Autodesk Fusion 360 part; units mm, degrees
sketch "Bottom Access Panel" plane through (0, 0, 0) normal (0, 1, 0) x (1, 0, 0)
  line L0 (0, 0) -> (140, 0)
  line L1 (140, 0) -> (140, -140)
  line L2 (140, -140) -> (0, -140)
  line L3 (0, -140) -> (0, 0)
  dimension "d1" = 140
  dimension "d2" = 140
extrude "Extrude1" add sketch "Bottom Access Panel" along normal blind 6
fillet "Fillet1" radius 8 4 edges at (0, 3, 140) (140, 3, 140) (140, 3, 0) (0, 3, 0)
sketch "Magnet Holes" plane through (0, 0, 0) normal (0, 1, 0) x (1, 0, 0)
  arc A0 (8, 0) -> (0, -8) centre (8, -8) ccw
  line L0 (8, 0) -> (132, 0)
  arc A1 (140, -8) -> (132, 0) centre (132, -8) ccw
  line L1 (140, -8) -> (140, -132)
  arc A2 (132, -140) -> (140, -132) centre (132, -132) ccw
  line L2 (132, -140) -> (8, -140)
  arc A3 (0, -132) -> (8, -140) centre (8, -132) ccw
  line L3 (0, -132) -> (0, -8)
  circle A4 centre (10, -130) radius 2.75
  circle A5 centre (130, -130) radius 2.75
  circle A6 centre (10, -10) radius 2.75
  circle A7 centre (130, -10) radius 2.75
  dimension "d20" = 5.5
  dimension "d21" = 5.5
  dimension "d22" = 5.5
  dimension "d23" = 5.5
  dimension "d24" = 10
  dimension "d25" = 10
  dimension "d26" = 10
  dimension "d27" = 10
  dimension "d28" = 10
  dimension "d29" = 10
  dimension "d30" = 10
  dimension "d31" = 10
extrude "Extrude3" cut sketch "Magnet Holes" along normal blind 1.5 contours A4 | A5 | A6 | A7
equation "mdfThickness = 6 mm"
equation "d4 = mdfThickness"
equation "filletRadius = 8 mm"
equation "d15 = filletRadius"
Part model, mm, in its own coordinate system. A direction names the side the tool comes from. Round coordinates to 2 decimals unless told otherwise and drop trailing zeros. Write each loop counter-clockwise with the first axis right and the second up, starting at its lowest first coordinate (ties: lowest second). Pieces come first, ordered by that corner, then holes.
Item 1: Probe L1, parallel to Z at x = 130, y = 1.15. List the from-to ranges inside material, lowest first.
Results:
L1: z = 0 to 7.25, 12.75 to 127.25, 132.75 to 140
Item 2: Which spindle directions (+Z, -Z, +X, -X, +Y, -Y) get a long thin tool onto all of the face, cutting with end or side? Do faces 1 (the cylindrical face through (137.594, 3.042, 137.719)), 2 (the flat face through (10, 1.5, 10)). Say none if no direction does.
Results:
face 1: +Z, +X, +Y, -Y
face 2: -Y
Item 3: Two-plate mould, pull along X, no slides. Class faces 3 (the flat face through (130, 1.5, 130)), 4 (the cylindrical face through (131.27, 0.74, 127.56)), 5 (the flat face through (140, 3, 69)), 6 (the flat face through (69, 0, 69)): +X half, -X half, draft (parallel to the pull), parting line (faces both ways), or undercut.
Results:
face 3: undercut
face 4: undercut
face 5: +X half
face 6: draft
Item 4: Drop a flat-ended pin along its axis: pin 1 Ø1.6 at (x, z) = (9.5, 9) entering from -Y. Give the stop position or say it passes through.
Results:
pin 1: stops at y = 1.5
Item 5: Cut at B-B, the plane z = 10. Give the cut face in (x, y).
Results:
outline: (0, 0) - (7.25, 0) - (7.25, 1.5) - (12.75, 1.5) - (12.75, 0) - (127.25, 0) - (127.25, 1.5) - (132.75, 1.5) - (132.75, 0) - (140, 0) - (140, 6) - (0, 6) - close
Item 6: Cut at A-A, the plane x = 130. Give the cut face in (y, z), plus the area to 4 significant figures.
Results:
outline: (0, 0) - (6, 0) - (6, 140) - (0, 140) - (0, 132.75) - (1.5, 132.75) - (1.5, 127.25) - (0, 127.25) - (0, 12.75) - (1.5, 12.75) - (1.5, 7.25) - (0, 7.25) - close
area: 823.5 mm2
